The model under review builds one solid part; all positions refer to its coordinate system, in mm. Face numbers are marked on the shaded views. A direction names the side the tool comes from. Give positions to 0.01 mm unless a question says otherwise; leave off trailing zeros. Write each loop counter-clockwise with the first axis right and the second up, starting at its lowest first coordinate (ties: lowest second). Pieces come first, ordered by that corner, then holes. Notation, with made-up numbers: M 20,33.5 L 56,33.5 A24 cw 56,62.5 Z; hole C 48.25,-2.75 d3. An arc over 180 degrees is marked long. Write each question's results on one line, items separated by ' | '. Start each with the question number.
from build123d import *

# Parameters (mm, degrees)
SKETCH2_R           = 4
BOSS_EXTRUDE1_DEPTH = 1
SKETCH4_R           = 1
CUT_EXTRUDE1_DEPTH  = 2.5
SKETCH6_R           = 1.25
SKETCH6_R_2         = 1
BOSS_EXTRUDE4_DEPTH = 2
SKETCH5_R           = 0.25
CUT_EXTRUDE2_DEPTH  = 2
CIRPATTERN1_COUNT   = 5


with BuildPart() as part:
    # Sketch2 → Boss-Extrude1 (new body)
    with BuildSketch(Plane(origin=(0, 0, 0), x_dir=(0, 0, -1), z_dir=(1, 0, 0))):
        Circle(SKETCH2_R)
    extrude(amount=-BOSS_EXTRUDE1_DEPTH)

    # Sketch4 → Cut-Extrude1 (cut)
    with BuildSketch(Plane(origin=(0, 0, 0), x_dir=(0, 0, -1), z_dir=(1, 0, 0))):
        Circle(SKETCH4_R)
    extrude(amount=-CUT_EXTRUDE1_DEPTH, mode=Mode.SUBTRACT)

    # Sketch6 → Boss-Extrude4 (add)
    with BuildSketch(Plane.ZY.offset(1)):
        with Locations(Location((0, 0, 0), (0, 0, 180))):
            Circle(SKETCH6_R)
        with Locations(Location((0, 0, 0), (0, 0, 180))):
            Circle(SKETCH6_R_2, mode=Mode.SUBTRACT)
    extrude(amount=BOSS_EXTRUDE4_DEPTH)

    # Sketch5 → Cut-Extrude2 (cut)
    with BuildSketch(Plane(origin=(0, 0, 0), x_dir=(0, 0, -1), z_dir=(1, 0, 0))):
        with Locations((0, 3)):
            Circle(SKETCH5_R)
    cut_extrude2 = extrude(amount=-CUT_EXTRUDE2_DEPTH, mode=Mode.SUBTRACT)

    # CirPattern1: Cut-Extrude2 ×5 about axis
    cirpattern1_axis = Axis((0, 0, 0), (1, 0, 0))
    for i in range(1, CIRPATTERN1_COUNT):
        add(cut_extrude2.rotate(cirpattern1_axis, i * 360 / CIRPATTERN1_COUNT), mode=Mode.SUBTRACT)


solid = part.part
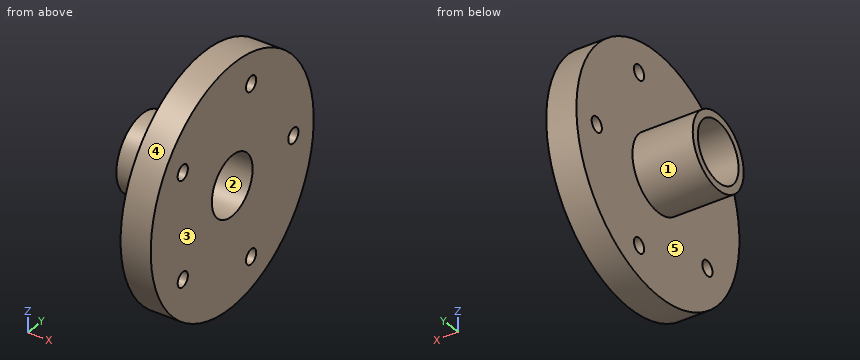
(1) Add section A-A (z = 0). State the section outline as (x, y) points.
(2) Wall thickness on L1, parallel to Z at x = -2.2, y = -0.5; L2, parallel to X at y = 0.25, z = 2.75; L3, parallel to Z at x = -0.95, y = -2.25: over which ranges is each line inside the solid? List them lowest first.
(3) Draft analysis for pull direction Y (two halves, no side actions). For the marked faces 1, 2 and 3, state which applies: pulls with the +Y half, pulls with the -Y half, needs draft (parallel to the pull), parting line crosses it, or undercut.
(4) Machinability: for the marked faces 4 and 5, which of the approach directions +Z, -Z, +X, -X, +Y, -Y give a long, thin tool a straight path to every point of the face, cutting with its end or side? Answer none if there is none.
(5) Add section C-C (z = 3). State the section outline as (x, y) points.
(6) Add section B-B (y = 0). State the section outline as (x, z) points.
(7) Add section D-D (x = -1.95). State the section outline as (y, z) points.
Calculated:
1) outline: M -3,-1.25 L -1,-1.25 L -1,-4 L 0,-4 L 0,-1 L -3,-1 Z; M -3,1 L 0,1 L 0,2.75 L -1,2.75 L -1,1.25 L -3,1.25 Z; M -1,3.25 L 0,3.25 L 0,4 L -1,4 Z
2) L1: z = -1.15 to -0.87, 0.87 to 1.15 | L2: x = -1 to 0 | L3: z = -3.31 to -1.94, -1.59 to 1.59, 1.94 to 3.31
3) face 1: parting line crosses it | face 2: undercut | face 3: needs draft
4) face 4: +X, -X | face 5: -X
5) outline: M -1,-2.65 L 0,-2.65 L 0,0.72 L -1,0.72 Z; M -1,1.13 L 0,1.13 L 0,2.65 L -1,2.65 Z
6) outline: M -3,-1.25 L -1,-1.25 L -1,-4 L 0,-4 L 0,-1 L -3,-1 Z; M -3,1 L 0,1 L 0,4 L -1,4 L -1,1.25 L -3,1.25 Z
7) outline: C 0,0 d2.5; hole C 0,0 d2
